Read the model definition and answer for the solid it produces. Units are mm, in the model's axes. A direction names the side the tool comes from. Give positions to 0.01 mm unless a question says otherwise; leave off trailing zeros. Write each loop counter-clockwise with the first axis right and the second up, starting at its lowest first coordinate (ties: lowest second). Pieces come first, ordered by that corner, then holes. Notation, with made-up numbers: M 55.5,77 L 105.5,77 A10 ccw 105.5,86 Z; hole C 30.25,49 d6. An arc over 180 degrees is marked long. Answer as CSV lines item,"result". Start each with the question number.
```python
from build123d import *

# Parameters (mm, degrees)
F0_R        = 2
F1_DEPTH    = 8
F2_R        = 3.5
F2_R_2      = 2
F3_DEPTH    = 0.5
F4_W        = 0.3
F4_H        = 3.9893038338
F5_DEPTH    = 15
F6_T1_DEPTH = 24.7839198555
F7_R        = 1
F8_W        = 1.6560796648
F8_H        = 0.4959646612
F8_W_2      = 1.2781426776
F8_H_2      = 0.4874281585
F8_W_3      = 1.2889747159
F8_H_3      = 0.4549305886
F8_W_4      = 0.7887214828
F8_H_4      = 0.3866125997
F8_W_5      = 1.2771316105
F8_H_5      = 0.5377400666
F9_DEPTH    = 0.3
F11_DEPTH   = 0.1
F13_DEPTH   = 0.1


# Not quite as in the source:
# - a fillet or chamfer that OpenCascade refuses, or shapes differently, is made with other operations: its cross-section is extruded or revolved along the edge and cut away or added


with BuildPart() as f1:
    # F0 (on Top) → F1 (new body)
    with BuildSketch(Plane.XY):
        Circle(F0_R)
    extrude(amount=F1_DEPTH)

    # F2 (on face) → F3 (join)
    with BuildSketch(Plane.XY.offset(8)):
        Circle(F2_R)
        Circle(F2_R_2, mode=Mode.SUBTRACT)
        Circle(F2_R_2)
    extrude(amount=F3_DEPTH)

    # F4 (on face) → F5 (join)
    with BuildSketch(Plane.XY.offset(8.5)):
        with Locations((0, -0.1216841047)):
            Rectangle(F4_W, F4_H)
    extrude(amount=F5_DEPTH)

    # F6: fillet of radius 5 on 1 edges, made by hand

    # F6_s2 → F6_t1 (cut)
    with BuildSketch(Plane.YZ.offset(-12.3919599278)):
        with BuildLine():
            ThreePointArc((-2.1163360216, 18.6032160289), (-0.9927700034, 21.7612628279), (1.8729678122, 23.5))
            Line((1.8729678122, 23.5), (-2.1163360216, 23.5))
            Line((-2.1163360216, 23.5), (-2.1163360216, 18.6032160289))
        make_face()
    extrude(amount=F6_T1_DEPTH, mode=Mode.SUBTRACT)

    # F7
    f7_edges = [f1.edges().sort_by_distance(p)[0] for p in [
        (-2, 0, 0),
    ]]
    fillet(f7_edges, radius=F7_R)

    # F8 (on face) → F9 (cut)
    with BuildSketch(Plane(origin=(-0.15, 0, 0), x_dir=(0, -1, 0), z_dir=(-1, 0, 0))):
        with Locations((2.2049986292, 19.7972180322)):
            Rectangle(F8_W, F8_H)
        with Locations((2.2229513852, 18.5654982924)):
            Rectangle(F8_W_2, F8_H_2)
        with Locations((1.5892958909, 20.9105657414)):
            Rectangle(F8_W_3, F8_H_3)
        with Locations((0.598409262, 21.9545691277)):
            Rectangle(F8_W_4, F8_H_4)
        with Locations((2.3904092959, 17.1525618061)):
            Rectangle(F8_W_5, F8_H_5)
    extrude(amount=-F9_DEPTH, mode=Mode.SUBTRACT)

    # F10 (on face) → F11 (cut)
    with BuildSketch(Plane(origin=(-0.15, 0, 0), x_dir=(0, -1, 0), z_dir=(-1, 0, 0))):
        with BuildLine():
            Line((-1.4041818934, 21.1293072328), (-1.4041818934, 9.1293072328))
            Line((-1.4041818934, 9.1293072328), (0.5958181066, 9.1293072328))
            Line((0.5958181066, 9.1293072328), (0.5958181066, 19.1293072328))
            ThreePointArc((0.5958181066, 19.1293072328), (0.010031669, 20.5435207952), (-1.4041818934, 21.1293072328))
        make_face()
    extrude(amount=-F11_DEPTH, mode=Mode.SUBTRACT)

    # F12 (on face) → F13 (cut)
    with BuildSketch(Plane.YZ.offset(0.15)):
        with BuildLine():
            Line((-0.5063290591, 9.1143995523), (1.4634948457, 9.1143995523))
            Line((1.4634948457, 9.1143995523), (1.4634948457, 21.1303744976))
            ThreePointArc((1.4634948457, 21.1303744976), (0.06882846, 20.5341063118), (-0.5063290591, 19.1306021597))
            Line((-0.5063290591, 19.1306021597), (-0.5063290591, 9.1143995523))
        make_face()
    extrude(amount=-F13_DEPTH, mode=Mode.SUBTRACT)


solid = f1.part
```
1. Find section C-C on y = 3. Determine the outline of the cut face in (x, z), then the cut area to 3 significant figures.
2. For faces 1 (the face through (0.15, -1, 16)), 2 (the face through (0, 0.5, 23)), 3 (the face through (0, 0, 0)), 4 (the face through (-0.15, -1, 16)), 5 (the face through (2, -2, 8)), determine the directions among +Z, -Z, +X, -X, +Y, -Y from which every point of the face is accessible in a straight line to the end or side of a thin tool.
3. Find section B-B on z = 4.25. Determine the outline of the cut face in (x, y).
4. Find section A-A on x = -2.25. Determine the outline of the cut face in (y, z), then the cut area to 3 significant figures.
5. Given pin 1 (1.5 mm diameter, centred on x = -2, y = -2, fed in from +Z); pin 2 (2 mm diameter, centred on y = 0.5, z = 18.5, fed in from +X); pin 3 (3.5 mm diameter, centred on x = 0, y = -1.5, fed in from +Z), each flat-ended and moving along its own axis, determine where each tip first touches the part or whether it passes through.
6. Find the intervals of material crossed by line 1 (Z direction, x = 0.5, y = 0.5); line 2 (Z direction, x = -2.25, y = 1); line 3 (X direction, y = -1.25, z = 9), in increasing order. Write a range as [from, to].
Computed:
1,outline,"M -1.8,8 L 1.8,8 L 1.8,8.5 L -1.8,8.5 Z"
1,area,"1.80 mm^2"
2,face 1,"+Z, +X, +Y, -Y"
2,face 2,"+Z, +X, -X, -Y"
2,face 3,"-Z, +X, -X, +Y, -Y"
2,face 4,"+Z, -X, +Y, -Y"
2,face 5,"-Z"
3,outline,"C 0,0 d4"
4,outline,"M -2.68,8 L 2.68,8 L 2.68,8.5 L -2.68,8.5 Z"
4,area,"2.68 mm^2"
5,pin 1,"stops at z = 8.5"
5,pin 2,"stops at x = 0.15"
5,pin 3,"stops at z = 22.85"
6,line 1,"z = [0, 8.5]"
6,line 2,"z = [8, 8.5]"
6,line 3,"x = [-0.15, 0.15]"
